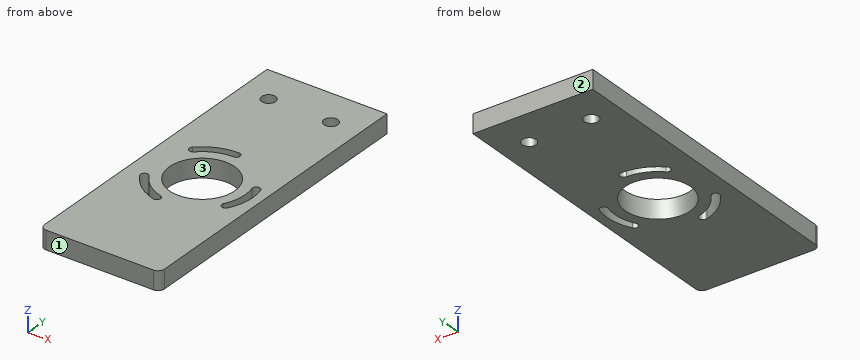
Autodesk Inventor part; units mm, degrees
ref_plane "YZ Plane" through (0, 0, 0) normal (1, 0, 0) x (0, 1, 0)
ref_plane "XZ Plane" through (0, 0, 0) normal (0, 1, 0) x (-1, 0, 0)
ref_plane "XY Plane" through (0, 0, 0) normal (0, 0, 1) x (1, 0, 0)
sketch "Sketch1" plane through (0, 0, 0) normal (0, 0, 1) x (1, 0, 0)
  circle A0 centre (0, -19.25) radius 10.5
  arc A1 (11.9852, -26.1697) -> (14.1148, -27.3992) centre (13.05, -26.7844) ccw
  arc A2 (-11.9852, -26.1697) -> (-14.1148, -27.3992) centre (-13.05, -26.7844) ccw
  arc A3 (0, -5.4107) -> (0, -2.9517) centre (0, -4.1812) ccw
  line L0 (0, -19.25) -> (14.5554, -15.3499) construction
  line L1 (0, -19.25) -> (13.05, -26.7844) construction
  line L2 (0, -19.25) -> (-10.6553, -8.5947) construction
  line L3 (0, -19.25) -> (0, -4.1812) construction
  line L4 (0, -19.25) -> (-3.9001, -33.8054) construction
  line L5 (0, -19.25) -> (-13.05, -26.7844) construction
  arc A4 (-4.2183, -34.993) -> (-3.5819, -32.6178) centre (-3.9001, -33.8054) ccw
  arc A5 (15.743, -15.0317) -> (13.3678, -15.6681) centre (14.5554, -15.3499) ccw
  arc A6 (-11.5247, -7.7253) -> (-9.7859, -9.4641) centre (-10.6553, -8.5947) ccw
  arc A7 (0, -2.9517) -> (-11.5247, -7.7253) centre (0, -19.25) ccw
  arc A8 (0, -5.4107) -> (-9.7859, -9.4641) centre (0, -19.25) ccw
  arc A9 (11.9852, -26.1697) -> (13.3678, -15.6681) centre (0, -19.25) ccw
  arc A10 (14.1148, -27.3992) -> (15.743, -15.0317) centre (0, -19.25) ccw
  arc A11 (-11.9852, -26.1697) -> (-3.5819, -32.6178) centre (0, -19.25) ccw
  arc A12 (-14.1148, -27.3992) -> (-4.2183, -34.993) centre (0, -19.25) ccw
  line L6 (19.25, -19.25) -> (19.25, 35.75)
  line L7 (-19.25, -19.25) -> (-19.25, 35.75)
  line L8 (19.25, 35.75) -> (-19.25, 35.75)
  circle A13 centre (-10, 23.75) radius 2.25
  circle A14 centre (10, 23.75) radius 2.25
  line L9 (10, 23.75) -> (-10, 23.75)
  line L10 (-19.25, -19.25) -> (-19.25, -62.25)
  line L11 (-17.25, -64.25) -> (17.25, -64.25)
  line L12 (19.25, -62.25) -> (19.25, -19.25)
  arc A15 (-19.25, -62.25) -> (-17.25, -64.25) centre (-17.25, -62.25) ccw
  arc A16 (17.25, -64.25) -> (19.25, -62.25) centre (17.25, -62.25) ccw
  point P0 (0, 0)
  point P1 (19.25, 30.75)
  point P2 (-19.25, -64.25)
  dimension "d0" = 21
  dimension "d1" = 45
  dimension "d2" = 45
  dimension "d3" = 45
  dimension "d4" = 2.459
  dimension "d5" = 2.459
  dimension "d6" = 2.459
  dimension "d7" = 2.459
  dimension "d8" = 2.459
  dimension "d9" = 2.459
  dimension "d11" = 55
  dimension "d21" = 4.5
  dimension "d22" = 12
  dimension "d23" = 4.5
  dimension "d24" = 20
  dimension "d25" = 9.25
  dimension "d26" = 38.5
  dimension "d27" = 45
  dimension "d28" = 2
extrude "Extrusion1" add sketch "Sketch1" along normal blind 6
equation "\"d8\" = d6"
equation "\"d9\" = d7"
equation "\"d23\" = d21"
equation "\"d25\" = -0.5 * d24 + 0.5 * d26"
properties part number "BaseC_7" material "PMMA Plastic"
Design review of the part built by this model. Coordinates are the model's own, in mm. Face numbers are marked on the shaded views. Coordinates: 2 decimals unless noted, no trailing zeros. Order: outer loops, then holes, each group sorted by start corner. A loop starts at its lowest first (then second) coordinate and runs counter-clockwise, first axis right, second up. Notation, with made-up numbers: (-35.5, 18.25) -> (10.5, 18.25) arc R22 ccw to (10.5, 50.25) -> close; hole circle Ø3 at (-11.5, -40). An arc over 180 degrees is marked (long way). Use one line per item in the form item = value. Start each with the question number.
(1) Add section B-B on y = 23.75. State the section outline as (x, z) points, plus the area to 3 significant figures.
(2) Add section A-A on y = -19.25. State the section outline as (x, z) points.
(3) Insertion check: pin 1 (5 mm diameter, centred on x = -4, y = 24.5, fed in from -Z). The pin has a flat end and moves straight along its axis. Give the tip position at first contact, or say it passes through.
(4) Add section C-C on z = 3.65. State the section outline as (x, y) points.
(5) The part is to be moulded in two halves that separate along Y. For the marked faces 1, 2 and 3, say which applies: +Y half, -Y half, draft (parallel to the pull), parting line (faces both ways), or undercut.
(6) For probe 1 along Y at (x, z) = (0, 2.8); probe 2 along X at (y, z) = (-24, 2.75); probe 3 along Y at (x, z) = (-4, 4.55), list the stretches that pass through material, from the lowest coordinate up.
Answer block:
q1.outline = (-19.25, 0) -> (-12.25, 0) -> (-12.25, 6) -> (-19.25, 6) -> close; (-7.75, 0) -> (7.75, 0) -> (7.75, 6) -> (-7.75, 6) -> close; (12.25, 0) -> (19.25, 0) -> (19.25, 6) -> (12.25, 6) -> close
q1.area = 177 mm²
q2.outline = (-19.25, 0) -> (-10.5, 0) -> (-10.5, 6) -> (-19.25, 6) -> close; (10.5, 0) -> (13.84, 0) -> (13.84, 6) -> (10.5, 6) -> close; (16.3, 0) -> (19.25, 0) -> (19.25, 6) -> (16.3, 6) -> close
q3.pin_1 = 0
q4.outline = (-19.25, -62.25) arc R2 ccw to (-17.25, -64.25) -> (17.25, -64.25) arc R2 ccw to (19.25, -62.25) -> (19.25, 35.75) -> (-19.25, 35.75) -> close; hole (-14.11, -27.4) arc R16.3 ccw to (-4.22, -34.99) arc R1.23 ccw to (-3.58, -32.62) arc R13.84 cw to (-11.99, -26.17) arc R1.23 ccw to start; hole circle Ø4.5 at (-10, 23.75); hole (-11.52, -7.73) arc R1.23 ccw to (-9.79, -9.46) arc R13.84 cw to (0, -5.41) arc R1.23 ccw to (0, -2.95) arc R16.3 ccw to start; hole circle Ø21 at (0, -19.25); hole circle Ø4.5 at (10, 23.75); hole (11.99, -26.17) arc R1.23 ccw to (14.11, -27.4) arc R16.3 ccw to (15.74, -15.03) arc R1.23 ccw to (13.37, -15.67) arc R13.84 cw to start
q5.face_1 = -Y half
q5.face_2 = +Y half
q5.face_3 = undercut
q6.probe_1 = -64.25 to -29.75, -8.75 to -5.41, -2.95 to 35.75
q6.probe_2 = -19.25 to -9.36, 9.36 to 13, 15.59 to 19.25
q6.probe_3 = -64.25 to -35.03, -32.5 to -28.96, -9.54 to -6, -3.45 to 35.75
